Solid Edge part; units mm, degrees
sketch "Sketch1" plane through (0, 0, 0) normal (0, -1, 0) x (1, 0, 0)
  circle A0 centre (0, 0) radius 24
extrude "Protrusion1" add sketch "Sketch1" along normal mid plane 300
sketch "Sketch2" plane through (0, 0, 0) normal (0, 0, 1) x (1, 0, 0)
  circle A0 centre (0, -56) radius 10
extrude "ExtrudedCutout_2" cut sketch "Sketch2" along normal blind 65.6181
sketch "Sketch3" plane through (0, 0, 0) normal (1, 0, 0) x (0, 1, 0)
  line L0 (49, 68.8622) -> (49, -45.9643)
extrude "ExtrudedCutout_3" cut sketch "Sketch3" along normal mid plane 174.551 material side at (0, 49.05, 11.4489)
sketch "Sketch4" plane through (0, 49, 0) normal (0, 1, 0) x (1, 0, 0)
  circle A0 centre (0, 0) radius 12.5
extrude "ExtrudedCutout_4" cut sketch "Sketch4" against normal blind 10
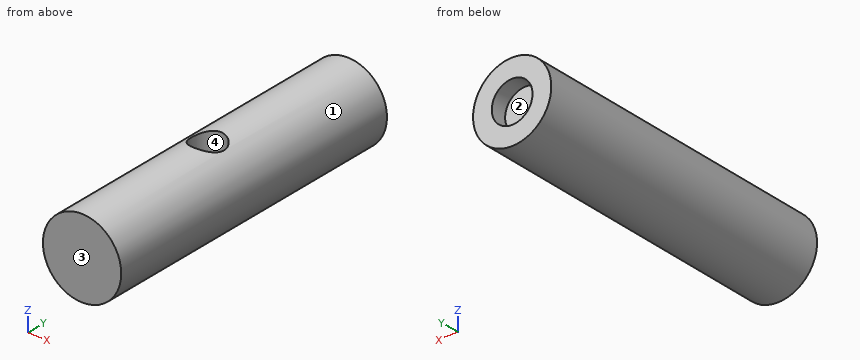
Verification items for the finished model (mm, model axes). Face numbers are marked on the shaded views. Coordinates: 2 decimals unless noted, no trailing zeros. Write each loop counter-clockwise with the first axis right and the second up, starting at its lowest first coordinate (ties: lowest second). Pieces come first, ordered by that corner, then holes. Notation, with made-up numbers: (-5.5, -18.5) - (32.5, -18.5) arc R17 cw to (32.5, -4.5) - close; hole circle Ø9 at (1.5, -27). An arc over 180 degrees is marked (long way). Answer as a JSON object with one key per item and string values.
(1) Cross-section at C-C on y = -35. Record the cut outline in (x, z), plus the area to 3 significant figures.
Report:
{"outline": "circle Ø48 at (0, 0)", "area": "1,810 mm^2"}
(2) Mould release check, pull along Y, two halves, no side actions. Record for the marked faces 1, 2, 3 and 4: pulls with the +Y half, pulls with the -Y half, needs draft (parallel to the pull), parting line crosses it, or undercut.
Report:
{"face 1": "needs draft", "face 2": "pulls with the +Y half", "face 3": "pulls with the -Y half", "face 4": "undercut"}
(3) Cross-section at A-A on z = 2.5. Record the cut outline in (x, y), plus the area to 3 significant figures.
Report:
{"outline": "(-23.87, -150) - (23.87, -150) - (23.87, 49) - (12.25, 49) - (12.25, 39) - (-12.25, 39) - (-12.25, 49) - (-23.87, 49) - close; hole circle Ø20 at (0, -56)", "area": "8,940 mm^2"}
(4) Thickness scan on line 1 along Z through (x, y) = (0, 45.75); line 2 along Y through (x, z) = (0, 8.5); line 3 along Y through (x, z) = (-8, 14). Record the ranges inside material, lowest first.
Report:
{"line 1": "-24 to -12.5, 12.5 to 24", "line 2": "-150 to -66, -46 to 39", "line 3": "-150 to -62, -50 to 49"}
(5) Cross-section at B-B on x = 0. Record the cut outline in (y, z).
Report:
{"outline": "(-150, -24) - (49, -24) - (49, -12.5) - (39, -12.5) - (39, 12.5) - (49, 12.5) - (49, 24) - (-46, 24) - (-46, 0) - (-66, 0) - (-66, 24) - (-150, 24) - close"}
(6) Cross-section at D-D on x = 8. Record the cut outline in (y, z), plus the area to 3 significant figures.
Report:
{"outline": "(-150, -22.63) - (49, -22.63) - (49, -9.6) - (39, -9.6) - (39, 9.6) - (49, 9.6) - (49, 22.63) - (-50, 22.63) - (-50, 0) - (-62, 0) - (-62, 22.63) - (-150, 22.63) - close", "area": "8,540 mm^2"}
(7) Gauge pin test, flat ends, axial feed: pin 1 Ø8 at (x, y) = (-10, -45.5) entering from -Z; pin 2 Ø10 at (y, z) = (24.5, -8) entering from -X; pin 3 Ø12 at (y, z) = (15, -11.5) entering from +X. Record the tip position at first contact, or that the pin passes through.
Report:
{"pin 1": "z = -23.24", "pin 2": "x = -23.81", "pin 3": "x = 23.36"}
